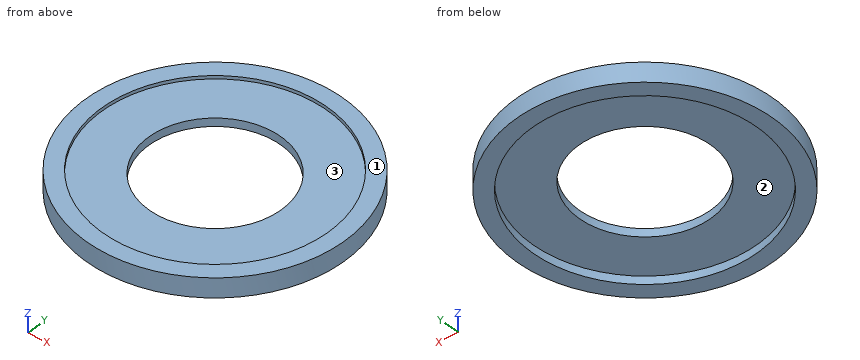
from build123d import *

# Parameters (mm, degrees)
OUTER_FLANGE_CONTACT_ANNULUS_ID8P2_START = 3
SKETCH1_R                                = 8
SKETCH1_R_2                              = 4.1
OUTER_FLANGE_CONTACT_ANNULUS_ID8P2_DEPTH = 0.5
M14X0P5_INTERNAL_THREAD_ENVELOPE_START   = 2.5
SKETCH2_R                                = 8
SKETCH2_R_2                              = 7
M14X0P5_INTERNAL_THREAD_ENVELOPE_DEPTH   = 1.2


with BuildPart() as part:
    # Sketch1 → Outer_Flange_Contact_Annulus_ID8p2 (new body)
    with BuildSketch(Plane.XY.offset(OUTER_FLANGE_CONTACT_ANNULUS_ID8P2_START)):
        Circle(SKETCH1_R)
        Circle(SKETCH1_R_2, mode=Mode.SUBTRACT)
    extrude(amount=OUTER_FLANGE_CONTACT_ANNULUS_ID8P2_DEPTH)

    # Sketch2 → M14x0p5_Internal_Thread_Envelope (add)
    with BuildSketch(Plane.XY.offset(M14X0P5_INTERNAL_THREAD_ENVELOPE_START)):
        Circle(SKETCH2_R)
        Circle(SKETCH2_R_2, mode=Mode.SUBTRACT)
    extrude(amount=M14X0P5_INTERNAL_THREAD_ENVELOPE_DEPTH)


solid = part.part
Work out the finished part from the listing and answer in its coordinate system (mm). Face numbers are marked on the shaded views. A direction names the side the tool comes from. Round coordinates to 2 decimals unless told otherwise and drop trailing zeros. Write each loop counter-clockwise with the first axis right and the second up, starting at its lowest first coordinate (ties: lowest second). Pieces come first, ordered by that corner, then holes.
1) A cutting plane is placed at C-C (z = 2.7). Give the vertices of the cut face in (x, y), plus the area to 3 significant figures.
2) Given pin 1 Ø1 at (x, y) = (4.5, -1) entering from -Z; pin 2 Ø7 at (x, y) = (-1.5, -0.5) entering from +Z, each flat-ended and moving along its own axis, determine where each tip first touches the part or whether it passes through.
3) A cutting plane is placed at A-A (y = 0). Give the vertices of the cut face in (x, z), plus the area to 3 significant figures.
4) Straight lines are drawn through the part: line 1 (Y direction, x = 0, z = 3.55); line 2 (Y direction, x = 0, z = 3.35); line 3 (Z direction, x = -3.75, y = 5.5). For each, find the intervals that lie inside material, in ascending order.
5) A cutting plane is placed at D-D (y = -6). Give the vertices of the cut face in (x, z).
6) A tool of negligible diameter and unlimited length cuts with its end or side. For the marked faces 1, 2 and 3, from which of +Z, -Z, +X, -X, +Y, -Y can it reach the whole face along a straight path? Write none if from no direction.
Completed:
1. outline: circle Ø16 at (0, 0); hole circle Ø14 at (0, 0)
1. area: 47.1 mm2
2. pin 1: stops at z = 3
2. pin 2: stops at z = 3.5
3. outline: (-8, 2.5) - (-7, 2.5) - (-7, 3) - (-4.1, 3) - (-4.1, 3.5) - (-7, 3.5) - (-7, 3.7) - (-8, 3.7) - close; (4.1, 3) - (7, 3) - (7, 2.5) - (8, 2.5) - (8, 3.7) - (7, 3.7) - (7, 3.5) - (4.1, 3.5) - close
3. area: 5.30 mm2
4. line 1: y = -8 to -7, 7 to 8
4. line 2: y = -8 to -4.1, 4.1 to 8
4. line 3: z = 3 to 3.5
5. outline: (-5.29, 2.5) - (-3.61, 2.5) - (-3.61, 3) - (3.61, 3) - (3.61, 2.5) - (5.29, 2.5) - (5.29, 3.7) - (3.61, 3.7) - (3.61, 3.5) - (-3.61, 3.5) - (-3.61, 3.7) - (-5.29, 3.7) - close
6. face 1: +Z, +X, -X, +Y, -Y
6. face 2: -Z
6. face 3: +Z
